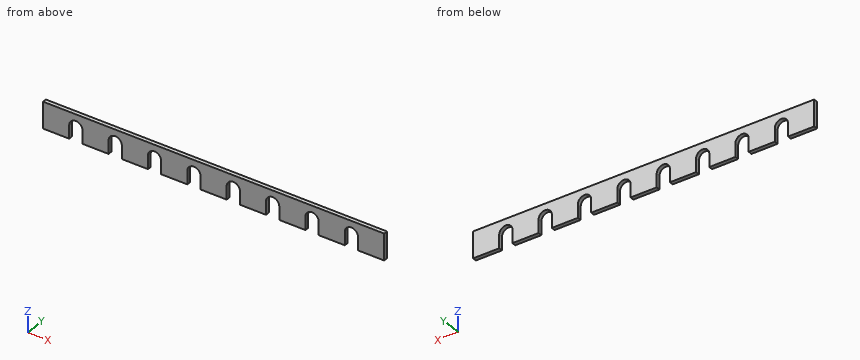
```python
from build123d import *

# Parameters (mm, degrees)
F1_DEPTH = 3


with BuildPart() as f1:
    # F0 (on Front) → F1 (new body)
    with BuildSketch(Plane.XZ):
        with BuildLine():
            Line((130, -10), (130, 10))
            Line((130, 10), (-130, 10))
            Line((-130, 10), (-130, -10))
            Line((-130, -10), (-110.05, -10))
            Line((-110.05, -10), (-110.05, 0))
            ThreePointArc((-110.05, 0), (-105, 5.05), (-99.95, 0))
            Line((-99.95, 0), (-99.95, -10))
            Line((-99.95, -10), (-80.05, -10))
            Line((-80.05, -10), (-80.05, 0))
            ThreePointArc((-80.05, 0), (-75, 5.05), (-69.95, 0))
            Line((-69.95, 0), (-69.95, -10))
            Line((-69.95, -10), (-50.05, -10))
            Line((-50.05, -10), (-50.05, 0))
            ThreePointArc((-50.05, 0), (-45, 5.05), (-39.95, 0))
            Line((-39.95, 0), (-39.95, -10))
            Line((-39.95, -10), (-20.05, -10))
            Line((-20.05, -10), (-20.05, 0))
            ThreePointArc((-20.05, 0), (-15, 5.05), (-9.95, 0))
            Line((-9.95, 0), (-9.95, -10))
            Line((-9.95, -10), (9.95, -10))
            Line((9.95, -10), (9.95, 0))
            ThreePointArc((9.95, 0), (15, 5.05), (20.05, 0))
            Line((20.05, 0), (20.05, -10))
            Line((20.05, -10), (39.95, -10))
            Line((39.95, -10), (39.95, 0))
            ThreePointArc((39.95, 0), (45, 5.05), (50.05, 0))
            Line((50.05, 0), (50.05, -10))
            Line((50.05, -10), (69.95, -10))
            Line((69.95, -10), (69.95, 0))
            ThreePointArc((69.95, 0), (75, 5.05), (80.05, 0))
            Line((80.05, 0), (80.05, -10))
            Line((80.05, -10), (99.95, -10))
            Line((99.95, -10), (99.95, 0))
            ThreePointArc((99.95, 0), (105, 5.05), (110.05, 0))
            Line((110.05, 0), (110.05, -10))
            Line((110.05, -10), (130, -10))
        make_face()
    extrude(amount=F1_DEPTH)


solid = f1.part
```
Input: part model. Units: mm. Frame: model coordinates. Give positions to 0.01 mm unless a question says otherwise; leave off trailing zeros. Write each loop counter-clockwise with the first axis right and the second up, starting at its lowest first coordinate (ties: lowest second). Pieces come first, ordered by that corner, then holes. Notation, with made-up numbers: (78.5, 74) - (127.5, 74) arc R20 ccw to (127.5, 105) - close; hole circle Ø10 at (84, 30). An arc over 180 degrees is marked (long way). Write item = value, one per line. Start each with the question number.
1) Cut plane A-A (z = -6.25). Give the number of separate pieces and of enclosed holes in the cut face, and give its area (3 significant figures).
2) Cut plane C-C (x = -13). Return loops of the section in (y, z), and give its area (3 significant figures).
3) Cut plane B-B (x = 45). Return loops of the section in (y, z).
4) Material intervals for L1, parallel to Z at x = 107.5, y = -0.55; L2, parallel to Z at x = -12, y = -1.3, sorted ascending. Write a range as [from, to].
Answers follow:
q1.separate_pieces = 9
q1.enclosed_holes = 0
q1.area = 538 mm^2
q2.outline = (-3, 4.64) - (0, 4.64) - (0, 10) - (-3, 10) - close
q2.area = 16.1 mm^2
q3.outline = (-3, 5.05) - (0, 5.05) - (0, 10) - (-3, 10) - close
q4.L1 = [4.39, 10]
q4.L2 = [4.06, 10]
